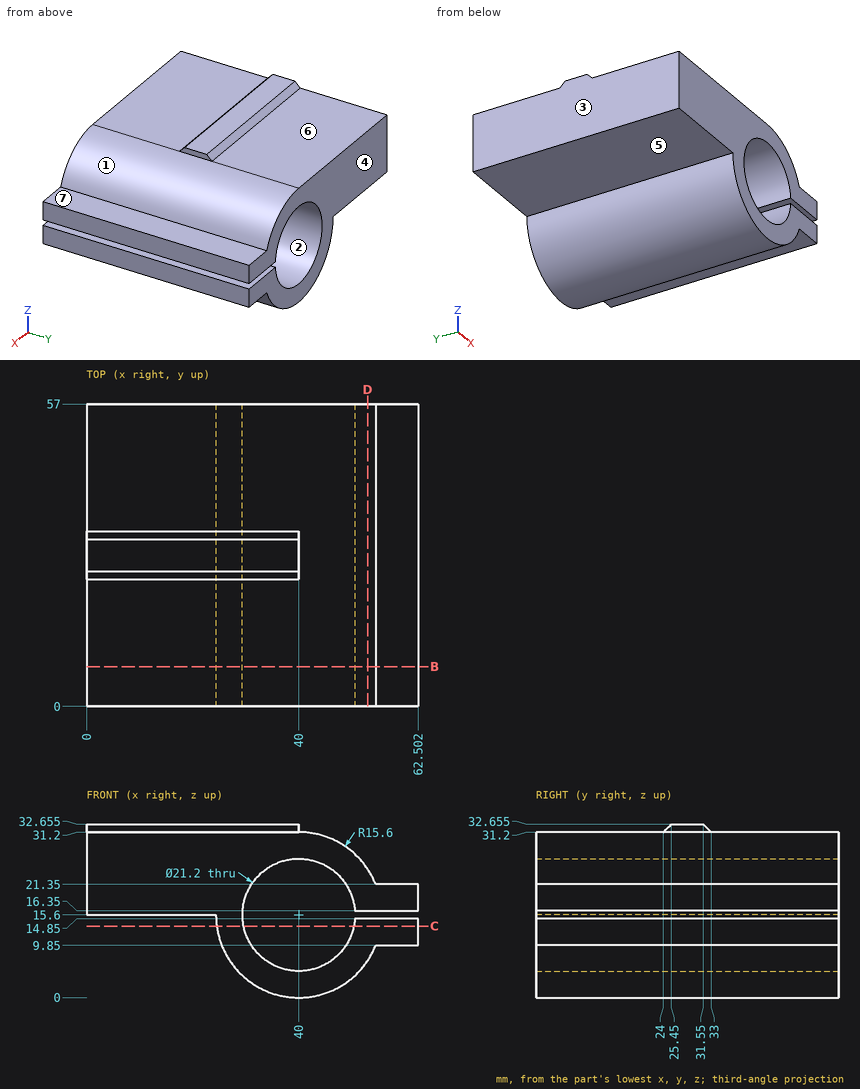
Check sheet for the drawn part. Datum: minimum x, y, z corner. Units: mm. A direction names the side the tool comes from. Coordinates: 2 decimals unless noted, no trailing zeros. Loops run counter-clockwise (first coordinate to the right, second up) from the corner with the lowest first, then second, coordinate; pieces in that order, holes last. Notation, with made-up numbers: (-25.5, 76) -> (-14.5, 76) arc R27 cw to (-14.5, 98) -> close; hole circle Ø5 at (16.25, 80.5). An arc over 180 degrees is marked (long way). Answer as a JSON object with one key per item and string values. Group by question number.
Item 1: Scan lines: probe 1 along Z at (x, y) = (40, 34.5); probe 2 along Z at (x, y) = (57, 49); probe 3 along X at (y, z) = (32.5, 14). Record each from-to range of solid material in increasing order.
Item 2: Sectioned sample at D-D on x = 53. Record the boundary of the cut face in (y, z).
Item 3: Mould release check, pull along X, two halves, no side actions. Record for the marked faces 1, 2, 3 and 4: +X half, -X half, draft (parallel to the pull), parting line (faces both ways), or undercut.
Item 4: Sectioned sample at B-B on y = 7.5. Record the boundary of the cut face in (x, z).
Item 5: Depth check by flat-ended pin: pin 1 (9 mm diameter, centred on x = 58.5, y = 25, fed in from +Z); pin 2 (19.5 mm diameter, centred on x = 7.5, y = 22.5, fed in from -Z); pin 3 (1 mm diameter, centred on y = 44, z = 8, fed in from +X). Enter the tip coordinate at first touch or a pass-through.
Item 6: Tool access check on the marked faces 5, 6 and 7. Record the directions out of +Z, -Z, +X, -X, +Y, -Y that give a thin tool (end or side, any length) a straight path to the whole face; none if there is none.
Item 7: Sectioned sample at C-C on z = 13.5. Record the boundary of the cut face in (x, y).
Evaluation:
{
 "1": {"probe 1": "z = 0 to 5, 26.2 to 31.2", "probe 2": "z = 9.85 to 14.85, 16.35 to 21.35", "probe 3": "x = 24.48 to 29.52, 50.48 to 62.5"},
 "2": {"outline": "(0, 6.98) -> (57, 6.98) -> (57, 14.85) -> (0, 14.85) -> close; (0, 16.35) -> (57, 16.35) -> (57, 24.22) -> (0, 24.22) -> close"},
 "3": {"face 1": "+X half", "face 2": "undercut", "face 3": "-X half", "face 4": "draft"},
 "4": {"outline": "(0, 15.6) -> (24.4, 15.6) arc R15.6 ccw to (54.5, 9.85) -> (62.5, 9.85) -> (62.5, 14.85) -> (50.57, 14.85) arc R10.6 cw (long way) to (50.57, 16.35) -> (62.5, 16.35) -> (62.5, 21.35) -> (54.5, 21.35) arc R15.6 ccw to (40, 31.2) -> (0, 31.2) -> close"},
 "5": {"pin 1": "stops at z = 22.48", "pin 2": "stops at z = 15.6", "pin 3": "stops at x = 53.89"},
 "6": {"face 5": "-Z, -X, +Y, -Y", "face 6": "+Z, +X, -X, +Y", "face 7": "+Z, +X, +Y, -Y"},
 "7": {"outline": "(24.54, 0) -> (29.61, 0) -> (29.61, 57) -> (24.54, 57) -> close; (50.39, 0) -> (62.5, 0) -> (62.5, 57) -> (50.39, 57) -> close"}
}
